Autodesk Inventor part; units mm, degrees
ref_plane "YZ Plane" through (0, 0, 0) normal (1, 0, 0) x (0, 1, 0)
ref_plane "XZ Plane" through (0, 0, 0) normal (0, 1, 0) x (-1, 0, 0)
ref_plane "XY Plane" through (0, 0, 0) normal (0, 0, 1) x (1, 0, 0)
sketch "Sketch1" plane through (0, 0, 0) normal (0, 0, 1) x (1, 0, 0)
  line L0 (0, 0) -> (0, 2.413)
  line L1 (0, 2.413) -> (-4.826, 2.413)
  line L2 (-4.826, 2.413) -> (-4.826, 3.175)
  line L3 (-4.826, 3.175) -> (-11.176, 3.175)
  line L4 (-11.176, 3.175) -> (-11.176, 3.81)
  line L5 (-11.176, 3.81) -> (-9.906, 3.81)
  line L6 (-9.906, 3.81) -> (-9.906, 3.429)
  line L7 (-9.906, 3.429) -> (0, 3.683)
  line L8 (0, 3.683) -> (0, 4.953)
  line L9 (0, 4.953) -> (1.778, 4.953)
  line L10 (1.778, 4.953) -> (1.778, 3.683)
  line L11 (1.778, 3.683) -> (11.43, 3.683)
  line L12 (11.43, 3.683) -> (11.43, 3.175)
  line L13 (11.43, 3.175) -> (10.16, 3.175)
  line L14 (10.16, 3.175) -> (10.16, 2.413)
  line L15 (10.16, 2.413) -> (1.778, 2.413)
  line L16 (1.778, 0) -> (0, 0)
  line L17 (1.778, 2.413) -> (1.778, 0)
  dimension "d0" = 8.382
  dimension "d2" = 0.508
  dimension "d3" = 0.762
  dimension "d4" = 1.27
  dimension "d5" = 1.778
  dimension "d6" = 2.413
  dimension "d7" = 0.254
  dimension "d8" = 1.27
  dimension "d9" = 1.27
  dimension "d10" = 1.27
  dimension "d11" = 4.826
  dimension "d12" = 6.35
  dimension "d13" = 0.635
  dimension "d15" = 0.762
revolve "Revolution1" add sketch "Sketch1" angle 360 about axis through (1.778, 0, 0) along (-1, 0, 0)
sketch "Sketch4" plane through (-11.176, 0, 0) normal (-1, 0, 0) x (0, 0, 1)
  line L0 (-0.508, 5.08) -> (0.508, 5.08)
  line L1 (0.508, 5.08) -> (0.508, -20.32)
  line L2 (0.508, -20.32) -> (-0.508, -20.32)
  line L3 (-0.508, -20.32) -> (-0.508, 5.08)
  point P0 (0, 0)
  point P1 (0, 4.442)
  dimension "d18" = 1.016
  dimension "d19" = 0.508
  dimension "d21" = 0
  dimension "d22" = 25.4
extrude "Extrusion1" cut sketch "Sketch4" against normal blind 5.08
properties part number "AxelDE" material "Polycarbonate, Clear"
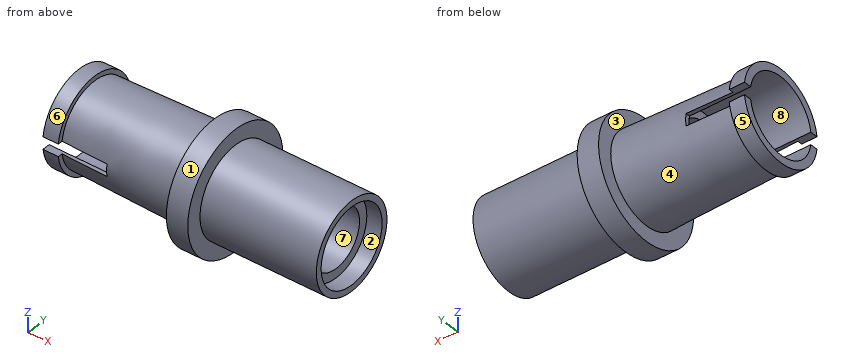
Geometry: final body of the model. Coordinates: model frame, mm. Face numbers are marked on the shaded views. A direction names the side the tool comes from. Round coordinates to 2 decimals unless told otherwise and drop trailing zeros. Write each loop counter-clockwise with the first axis right and the second up, starting at its lowest first coordinate (ties: lowest second). Pieces come first, ordered by that corner, then holes. Notation, with made-up numbers: (56.5, -34.5) -> (101.5, -34.5) arc R15 cw to (101.5, -14.5) -> close; hole circle Ø6 at (85, -27). An arc over 180 degrees is marked (long way). Return JSON: item names as keys, results as strings.
Q1. Set-up query: the marked faces 4, 5, 6, 7 and 8. Return all of +Z, -Z, +X, -X, +Y, -Y with unobstructed straight access to the full face (end or side cutting, diameter ignored); none if empty.
From the geometry:
{"face 4": "none", "face 5": "-Z, -X", "face 6": "+Z, -X", "face 7": "+X", "face 8": "-X"}
Q2. Section B-B on x = 7.25. Return the cut outline in (y, z).
From the geometry:
{"outline": "circle Ø7.37 at (0, 0); hole circle Ø4.83 at (0, 0)"}
Q3. Mould query, pull axis Y, two halves, no side actions, for the marked faces 1, 2 and 3. Classes: +Y half, -Y half, draft (parallel to the pull), parting line (faces both ways), or undercut.
From the geometry:
{"face 1": "parting line", "face 2": "undercut", "face 3": "draft"}
Q4. Section D-D on x = -1.5. Return the cut outline in (y, z).
From the geometry:
{"outline": "circle Ø7.29 at (0, 0); hole circle Ø4.83 at (0, 0)"}
Q5. Section A-A on z = 0. Return the cut outline in (x, y) (3 decimals).
From the geometry:
{"outline": "(-6.096, -3.527) -> (0, -3.683) -> (0, -4.953) -> (1.778, -4.953) -> (1.778, -3.683) -> (11.43, -3.683) -> (11.43, -3.175) -> (10.16, -3.175) -> (10.16, -2.413) -> (1.778, -2.413) -> (1.778, 2.413) -> (10.16, 2.413) -> (10.16, 3.175) -> (11.43, 3.175) -> (11.43, 3.683) -> (1.778, 3.683) -> (1.778, 4.953) -> (0, 4.953) -> (0, 3.683) -> (-6.096, 3.527) -> (-6.096, 3.175) -> (-4.826, 3.175) -> (-4.826, 2.413) -> (0, 2.413) -> (0, -2.413) -> (-4.826, -2.413) -> (-4.826, -3.175) -> (-6.096, -3.175) -> close"}
Q6. Ray query, line 1 (Z direction, x = 5.75, y = 0); line 2 (X direction, y = -0.5, z = 4); line 3 (Z direction, x = -1.65, y = 0). Return the intervals inside material, ascending.
From the geometry:
{"line 1": "-3.68 to -2.41, 2.41 to 3.68", "line 2": "0 to 1.78", "line 3": "-3.64 to -2.41, 2.41 to 3.64"}
Q7. First-contact query: pin 1 Ø3 at (x, z) = (6.5, 0.5) entering from -Y; pin 2 Ø2.5 at (y, z) = (0.5, -0.5) entering from +X; pin 3 Ø3 at (x, y) = (-7, -2.5) entering from +Z. Flat tips, straight axial feed; report the tip coordinate or a pass-through.
From the geometry:
{"pin 1": "y = -3.68", "pin 2": "x = 1.78", "pin 3": "z = 3.36"}
